from build123d import *

# Parameters (mm, degrees)
F0_R     = 5
F1_DEPTH = 10
F2_R     = 2.5
F3_DEPTH = 15


with BuildPart() as f1:
    # F0 (on Front) → F1 (new body)
    with BuildSketch(Plane.XZ):
        with BuildLine():
            ThreePointArc((0, 5), (1.464466, 1.464466), (5, 0))
            Line((5, 0), (195, 0))
            ThreePointArc((195, 0), (198.535534, 1.464466), (200, 5))
            Line((200, 5), (200, 10))
            ThreePointArc((200, 10), (198.535534, 13.535534), (195, 15))
            Line((195, 15), (5, 15))
            ThreePointArc((5, 15), (1.464466, 13.535534), (0, 10))
            Line((0, 10), (0, 5))
        make_face()
        with Locations((7.767204, 7.5)):
            Circle(F0_R, mode=Mode.SUBTRACT)
        with Locations((80, 7.5)):
            Circle(F0_R, mode=Mode.SUBTRACT)
    extrude(amount=F1_DEPTH)

    # F2 (on face) → F3 (join)
    with BuildSketch(Plane.XZ.offset(10)):
        with Locations((195.353363, 7.5)):
            Circle(F2_R)
    extrude(amount=F3_DEPTH)


solid = f1.part
For this review, take the finished solid that the model builds, in its own axes (mm). A direction names the side the tool comes from. Round coordinates to 2 decimals unless told otherwise and drop trailing zeros. Loops run counter-clockwise (first coordinate to the right, second up) from the corner with the lowest first, then second, coordinate; pieces in that order, holes last. Notation, with made-up numbers: (38.25, -16.75) - (61.25, -16.75) arc R20 cw to (61.25, 15.25) - close; hole circle Ø11 at (-10, 24.25). An arc over 180 degrees is marked (long way). Answer as CSV lines item,"result".
(1) Consider section A-A on z = 7.5. Give the boundary of the cut face in (x, y), then the cut area to 4 significant figures.
Checked values:
outline,"(0, -10) - (2.77, -10) - (2.77, 0) - (0, 0) - close; (12.77, -10) - (75, -10) - (75, 0) - (12.77, 0) - close; (85, -10) - (192.85, -10) - (192.85, -25) - (197.85, -25) - (197.85, -10) - (200, -10) - (200, 0) - (85, 0) - close"
area,"1,875 mm2"
(2) Insertion check: P1, Ø3, axis at y = -15.5, z = 9, coming from the -X side; P2, Ø6, axis at x = 52, z = 6, coming from the -Y side; P3, Ø1, axis at y = -7, z = 11, coming from the -X side. Each pin has a flat end and moves straight along its axis. Give the tip position at first contact, or say it passes through.
Checked values:
P1,"stops at x = 192.85"
P2,"stops at y = -10"
P3,"stops at x = 0.03"
(3) Wall thickness on line 1 (X direction, y = -3.75, z = 5); line 2 (Z direction, x = 80, y = -3); line 3 (Y direction, x = 44.5, z = 12.25): over which ranges is each line inside the solid? List them lowest first.
Checked values:
line 1,"x = 0 to 3.44, 12.1 to 75.67, 84.33 to 200"
line 2,"z = 0 to 2.5, 12.5 to 15"
line 3,"y = -10 to 0"
(4) Consider section D-D on x = 187. Give the boundary of the cut face in (y, z).
Checked values:
outline,"(-10, 0) - (0, 0) - (0, 15) - (-10, 15) - close"
(5) Consider section C-C on y = -7. Give the boundary of the cut face in (x, z).
Checked values:
outline,"(0, 5) arc R5 ccw to (5, 0) - (195, 0) arc R5 ccw to (200, 5) - (200, 10) arc R5 ccw to (195, 15) - (5, 15) arc R5 ccw to (0, 10) - close; hole circle Ø10 at (7.77, 7.5); hole circle Ø10 at (80, 7.5)"
(6) Consider section B-B on x = 80. Give the boundary of the cut face in (y, z), then the cut area to 3 significant figures.
Checked values:
outline,"(-10, 0) - (0, 0) - (0, 2.5) - (-10, 2.5) - close; (-10, 12.5) - (0, 12.5) - (0, 15) - (-10, 15) - close"
area,"50.0 mm2"
(7) Tool access review of faces 4 (the face through (193.37, -17.4, 5.98)), 5 (the face through (2, -5, 14)): name each direction out of +Z, -Z, +X, -X, +Y, -Y from which nothing blocks a thin tool from reaching the whole face with its end or side.
Checked values:
face 4,"-Y"
face 5,"+Z, -X, +Y, -Y"
(8) Mouldability with a two-part tool opening along Z and no side actions: class faces 1 (the face through (99, 0, 8)), 2 (the face through (199, -5, 13)), 3 (the face through (84.619, -4.93, 5.585)) as +Z half, -Z half, draft (parallel to the pull), parting line (faces both ways), or undercut.
Checked values:
face 1,"draft"
face 2,"+Z half"
face 3,"undercut"
